from build123d import *

# Parameters (mm, degrees)
F2_R = 14.7170458762
F3_R = 5.08
F4_T = -2.54


with BuildPart() as f1:
    # F0 (on Front) → F1 (revolve)
    with BuildSketch(Plane.XZ):
        Polygon((0, -76.023183763), (0, 66.5910243988), (-15.4687426984, 66.5910243988), (-15.4687426984, 62.4408759177), (-11.3185923547, 62.4408759177), (-11.3185923547, 34.8989777267), (-30.9374798089, 26.9759688526), (-30.9374798089, -76.023183763), align=None)
    revolve(axis=Axis((0, 0, -4.7160796821), (0, 0, -1)))

    # F2
    f2_edges = [f1.edges().sort_by_distance(p)[0] for p in [
        (30.93748, 0, 26.975969),
        (11.318592, 0, 34.898978),
    ]]
    fillet(f2_edges, radius=F2_R)

    # F3
    f3_edges = [f1.edges().sort_by_distance(p)[0] for p in [
        (30.93748, 0, -76.023184),
    ]]
    fillet(f3_edges, radius=F3_R)

    # F4
    f4_openings = [f1.faces().sort_by_distance(p)[0] for p in [
        (0, 0, 66.591024),
    ]]
    offset(amount=F4_T, openings=f4_openings, kind=Kind.INTERSECTION)


solid = f1.part
The model under review builds one solid part; all positions refer to its coordinate system, in mm. A direction names the side the tool comes from. Coordinates: 2 decimals unless noted, no trailing zeros. Write each loop counter-clockwise with the first axis right and the second up, starting at its lowest first coordinate (ties: lowest second). Pieces come first, ordered by that corner, then holes. Notation, with made-up numbers: (-6, 25.5) - (23, 25.5) arc R14 cw to (23, 50.5) - close; hole circle Ø5 at (21, -34). An arc over 180 degrees is marked (long way). Answer as a JSON object with one key per item and string values. Group by question number.
1. To check wall thickness, follow probe 1 along Y at (x, z) = (0, -3); probe 2 along Z at (x, y) = (20.5, 2). State the ranges of each line that lie inside material, in increasing order.
2. Add section A-A (z = -51). Give the boundary of the cut face in (x, y).
3. Add section B-B (z = 55.5). Give the boundary of the cut face in (x, y).
4. Mouldability with a two-part tool opening along Z and no side actions: class faces 1 (the face through (0, 0, -73.483)), 2 (the face through (0, 0, -76.023)), 3 (the face through (-6.95, 10.9, 65.77)), 4 (the face through (8.34, 7.65, 53.51)) as pulls with the +Z half, pulls with the -Z half, needs draft (parallel to the pull), parting line crosses it, or undercut.
5. Machinability: for faces 5 (the face through (6.16, -27.72, -27.56)), 6 (the face through (-8.32, 13.04, 64.49)), 7 (the face through (-29.51, 9.29, -27.56)), which of the approach directions +Z, -Z, +X, -X, +Y, -Y give a long, thin tool a straight path to every point of the face, cutting with its end or side? Answer none if there is none.
6. Clearance check with flat-ended pins moving along their axes: pin 1 Ø1 at (y, z) = (2.5, -56.5) entering from -X; pin 2 Ø6 at (x, y) = (-7.5, 23.5) entering from +Z; pin 3 Ø4 at (y, z) = (-7, -33) entering from -X; pin 4 Ø20.5 at (x, y) = (-4, -5.5) entering from +Z. State where each tip first meets the part, or that it passes through.
Findings:
{
 "1": {"probe 1": "-30.94 to -28.4, 28.4 to 30.94", "probe 2": "-76.02 to -73.48, 28.41 to 31.15"},
 "2": {"outline": "circle Ø61.87 at (0, 0); hole circle Ø56.79 at (0, 0)"},
 "3": {"outline": "circle Ø22.64 at (0, 0); hole circle Ø17.56 at (0, 0)"},
 "4": {"face 1": "undercut", "face 2": "pulls with the -Z half", "face 3": "needs draft", "face 4": "undercut"},
 "5": {"face 5": "none", "face 6": "+Z", "face 7": "+Z, -Z"},
 "6": {"pin 1": "x = -30.87", "pin 2": "z = 30.72", "pin 3": "x = -30.53", "pin 4": "z = 66.59"}
}
